Here's how the part is built. I have some questions about the finished solid (model axes, mm). Coordinates: 2 decimals unless noted, no trailing zeros. Write each loop counter-clockwise with the first axis right and the second up, starting at its lowest first coordinate (ties: lowest second). Pieces come first, ordered by that corner, then holes.
Item 1: I want a section at C-C (z = -8). Count the separate pieces of the cut face and the enclosed holes in it, and give its area (3 significant figures).
Item 2: I want a section at B-B (y = -2.5). Please give me the cut outline in (x, z).
Item 3: If we mould it in two halves opening along Z, with no side actions, what happens to faces 1 (the face through (23, 0, 0)), 2 (the face through (23, 3.175, -10)), 3 (the face through (6.87, -0.06, -7.64)), 4 (the face through (23, 0, -19.05))? For each: pulls with the +Z half, pulls with the -Z half, needs draft (parallel to the pull), parting line crosses it, or undercut.
Item 4: I want a section at A-A (x = 40.64). Please give me the cut outline in (y, z) (3 decimals), and give its area (3 significant figures).
Item 5: Please list where these lines run through material, in increasing order: line 1 (Z direction, x = 5.08, y = 0.75); line 2 (X direction, y = -1.25, z = -8).
from build123d import *

# Parameters (mm, degrees)
SKETCH1_W                      = 45.72
SKETCH1_H                      = 19.05
BOSS_EXTRUDE1_DEPTH            = 3.175
M4_CLEARANCE_HOLE1_D           = 4.5
M4_CLEARANCE_HOLE1_CSINK_D     = 4.55
M4_CLEARANCE_HOLE1_CSINK_ANGLE = 90


with BuildPart() as part:
    # Sketch1 → Boss-Extrude1 (new, symmetric)
    with BuildSketch(Plane(origin=(0, 0, 0), x_dir=(1, 0, 0), z_dir=(0, 1, 0))):
        with Locations((22.86, 9.525)):
            Rectangle(SKETCH1_W, SKETCH1_H)
    extrude(amount=BOSS_EXTRUDE1_DEPTH, both=True)

    # M4 Clearance Hole1 (through all)
    with Locations(Plane(origin=(0, 3.175, 0), x_dir=(1, 0, 0), z_dir=(0, 1, 0))):
        with Locations((5.08, 9.005429498), (40.64, 9.005429498)):
            CounterSinkHole(M4_CLEARANCE_HOLE1_D / 2, M4_CLEARANCE_HOLE1_CSINK_D / 2, counter_sink_angle=M4_CLEARANCE_HOLE1_CSINK_ANGLE)


solid = part.part
Answer:
1. separate pieces: 3
1. enclosed holes: 0
1. area: 239 mm2
2. outline: (0, -19.05) - (45.72, -19.05) - (45.72, 0) - (0, 0) - close; hole circle Ø4.5 at (5.08, -9.01); hole circle Ø4.5 at (40.64, -9.01)
3. face 1: pulls with the +Z half
3. face 2: needs draft
3. face 3: undercut
3. face 4: pulls with the -Z half
4. outline: (-3.175, -19.05) - (3.175, -19.05) - (3.175, -11.28) - (3.15, -11.255) - (-3.175, -11.255) - close; (-3.175, -6.755) - (3.15, -6.755) - (3.175, -6.73) - (3.175, 0) - (-3.175, 0) - close
4. area: 92.4 mm2
5. line 1: z = -19.05 to -11.26, -6.76 to 0
5. line 2: x = 0 to 3.07, 7.09 to 38.63, 42.65 to 45.72
